from build123d import *

# Parameters (mm, degrees)
BOSS_EXTRUDE1_DEPTH = 2.54
SKETCH2_R           = 2.8448
CUT_EXTRUDE1_DEPTH  = 5.08


with BuildPart() as part:
    # Sketch1 → Boss-Extrude1 (new body, symmetric)
    with BuildSketch(Plane.XY):
        with BuildLine():
            Line((-106.203198828, 123.8526304), (-153.956362537, 110.054547529))
            Line((-153.956362537, 110.054547529), (-150.972399128, 97.006641248))
            Line((-150.972399128, 97.006641248), (-106.007662429, 109.999019449))
            ThreePointArc((-106.007662429, 109.999019449), (-66.301425243, 87.590832017), (-50.567785145, 44.798721708))
            Line((-50.567785145, 44.798721708), (-50.567785145, 27.018721708))
            Line((-50.567785145, 27.018721708), (-35.327785145, 27.018721708))
            Line((-35.327785145, 27.018721708), (-35.327785145, 45.691652598))
            ThreePointArc((-35.327785145, 45.691652598), (-55.685055667, 98.44689574), (-106.203198828, 123.8526304))
        make_face()
    extrude(amount=BOSS_EXTRUDE1_DEPTH, both=True)

    # Sketch2 → Cut-Extrude1 (cut)
    with BuildSketch(Plane.XY.offset(2.54)):
        with Locations((-43.152202962, 34.412244361)):
            Circle(SKETCH2_R)
    extrude(amount=-CUT_EXTRUDE1_DEPTH, mode=Mode.SUBTRACT)


solid = part.part
The listing builds one solid part. Answer for the finished solid, in the listing's coordinates (mm). A direction names the side the tool comes from. Round coordinates to 2 decimals unless told otherwise and drop trailing zeros. Write each loop counter-clockwise with the first axis right and the second up, starting at its lowest first coordinate (ties: lowest second). Pieces come first, ordered by that corner, then holes. Notation, with made-up numbers: M -6.75,8.5 L 35.25,8.5 A15 ccw 35.25,19.5 Z; hole C 68.25,-3.75 d11. An arc over 180 degrees is marked long. Write each question's results on one line, items separated by ' | '. Start each with the question number.
Item 1: A cutting plane is placed at C-C on y = 76.5. Write down the section's boundary in (x, z).
Item 2: Flat-ended cylindrical pins translate along their axes: pin 1 Ø1 at (y, z) = (45, 1) entering from -X; pin 2 Ø1.5 at (x, z) = (-131, 2) entering from -Y; pin 3 Ø3 at (x, z) = (-79, -1) entering from +Y. Find the tip coordinate at first contact, or state that the pin passes through.
Item 3: Straight lines are drawn through the part: L1, parallel to X at y = 33, z = -1.35; L2, parallel to X at y = 40, z = 0.1; L3, parallel to Y at x = -98, z = -1.3. For each, find the intervals that lie inside material, in ascending order. Write a range as [from, to].
Item 4: A cutting plane is placed at A-A on y = 36. Write down the section's boundary in (x, z).
Item 5: A cutting plane is placed at D-D on x = -59.5. Write down the section's boundary in (y, z), and give its area (3 significant figures).
Item 6: For faces 4 (the face through (-50.568, 36, 0)), 5 (the face through (-43, 27.019, 0)), 6 (the face through (-128.805, 103.412, 0.036)), determine the directions among +Z, -Z, +X, -X, +Y, -Y from which every point of the face is accessible in a straight line to the end or side of a thin tool.
Item 7: A cutting plane is placed at B-B on z = 1.55. Write down the section's boundary in (x, y), and give its area (3 significant figures).
Item 8: For a pull along Y with two mould halves and no side action, classify faces 1 (the face through (-66.73, 88.09, 0.04)), 2 (the face through (-129.75, 117.05, 0.04)), 3 (the face through (-43.769, 31.635, 0.036)) as pulls with the +Y half, pulls with the -Y half, needs draft (parallel to the pull), parting line crosses it, or undercut.
Check sheet entries:
1) outline: M -58.67,-2.54 L -41.62,-2.54 L -41.62,2.54 L -58.67,2.54 Z
2) pin 1: x = -50.57 | pin 2: y = 102.56 | pin 3: y = 116.79
3) L1: [-50.57, -45.62], [-40.68, -35.33] | L2: [-50.57, -35.33] | L3: [108.18, 122.61]
4) outline: M -50.57,-2.54 L -45.51,-2.54 L -45.51,2.54 L -50.57,2.54 Z; M -40.79,-2.54 L -35.33,-2.54 L -35.33,2.54 L -40.79,2.54 Z
5) outline: M 77.97,-2.54 L 102.37,-2.54 L 102.37,2.54 L 77.97,2.54 Z | area: 124 mm²
6) face 4: +Z, -Z, -X, -Y | face 5: +Z, -Z, +X, -X, -Y | face 6: +Z, -Z, -Y
7) outline: M -153.96,110.05 L -150.97,97.01 L -106.01,110 A66.06 cw -50.57,44.8 L -50.57,27.02 L -35.33,27.02 L -35.33,45.69 A78.54 ccw -106.2,123.85 Z; hole C -43.15,34.41 d5.69 | area: 2,450 mm²
8) face 1: pulls with the -Y half | face 2: pulls with the +Y half | face 3: undercut
